from build123d import *

# Parameters (mm, degrees)
SKETCH_1_R          = 70
SKETCH_1_R_2        = 58
EXTRUDE_1_DEPTH     = 9
SKETCH_3_R          = 70
SKETCH_3_R_2        = 61
CUT_EXTRUDE_2_DEPTH = 3
CUT_EXTRUDE_3_DEPTH = 100.403219264
FILLET_1_R          = 10
CUT_EXTRUDE_6_DEPTH = 97.044388064
FILLET_7_R          = 3
SKETCH_6_R          = 1.5
CUT_EXTRUDE_4_DEPTH = 10
FILLET_9_R          = 5
EXTRUDE_START       = -1
SKETCH_9_R          = 58
SKETCH_9_R_2        = 56
EXTRUDE_2_DEPTH     = 1


with BuildPart() as part:
    # 草图1 → 凸台-拉伸1 (new body)
    with BuildSketch(Plane(origin=(0, 0, 0), x_dir=(1, 0, 0), z_dir=(0, 1, 0))):
        with Locations(Location((0, 0, 0), (0, 0, 270))):
            Circle(SKETCH_1_R)
        with Locations(Location((0, 0, 0), (0, 0, 270))):
            Circle(SKETCH_1_R_2, mode=Mode.SUBTRACT)
    extrude(amount=EXTRUDE_1_DEPTH)

    # 草图3 → 切除-拉伸2 (cut)
    with BuildSketch(Plane.XZ):
        with Locations(Location((0, 0, 0), (0, 0, 270))):
            Circle(SKETCH_3_R)
        with Locations(Location((0, 0, 0), (0, 0, 270))):
            Circle(SKETCH_3_R_2, mode=Mode.SUBTRACT)
    extrude(amount=-CUT_EXTRUDE_2_DEPTH, mode=Mode.SUBTRACT)

    # 草图4 → 切除-拉伸3 (cut, through all)
    with BuildSketch(Plane(origin=(0, 9, 0), x_dir=(1, 0, 0), z_dir=(0, 1, 0))):
        with BuildLine():
            Line((35.848527272, 51.197002768), (40.150350545, 57.3406431))
            ThreePointArc((40.150350545, 57.3406431), (0, 70), (-40.150350545, 57.3406431))
            Line((-40.150350545, 57.3406431), (-35.848527272, 51.197002768))
            ThreePointArc((-35.848527272, 51.197002768), (0, 62.5), (35.848527272, 51.197002768))
        make_face()
        with BuildLine():
            Line((51.197002768, 35.848527272), (57.3406431, 40.150350545))
            ThreePointArc((57.3406431, 40.150350545), (68.936542711, 12.155372437), (67.61480784, -18.117333157))
            Line((67.61480784, -18.117333157), (60.370364143, -16.176190319))
            ThreePointArc((60.370364143, -16.176190319), (61.550484563, 10.853011104), (51.197002768, 35.848527272))
        make_face()
        with BuildLine():
            Line((16.176190319, -60.370364143), (18.117333157, -67.61480784))
            ThreePointArc((18.117333157, -67.61480784), (-12.155372437, -68.936542711), (-40.150350545, -57.3406431))
            Line((-40.150350545, -57.3406431), (-35.848527272, -51.197002768))
            ThreePointArc((-35.848527272, -51.197002768), (-10.853011104, -61.550484563), (16.176190319, -60.370364143))
        make_face()
        with BuildLine():
            Line((-51.197002768, -35.848527272), (-57.3406431, -40.150350545))
            ThreePointArc((-57.3406431, -40.150350545), (-70, 0), (-57.3406431, 40.150350545))
            Line((-57.3406431, 40.150350545), (-51.197002768, 35.848527272))
            ThreePointArc((-51.197002768, 35.848527272), (-62.5, 0), (-51.197002768, -35.848527272))
        make_face()
    extrude(amount=-CUT_EXTRUDE_3_DEPTH, mode=Mode.SUBTRACT)

    # 圆角1
    # the kernel refuses this fillet: 10 mm, written as the material it adds along each edge
    with BuildSketch(Plane(origin=(-51.197002768, 9, 35.848527272), x_dir=(-0.8191520442890221, 0, 0.5735764363510029), z_dir=(0, -1, 0)), Plane(origin=(51.197002768, 9, -35.848527272), x_dir=(0.8191520442890228, 0, -0.5735764363510018), z_dir=(0, -1, 0)), Plane(origin=(-35.848527272, 9, -51.197002768), x_dir=(-0.5735764363510008, 0, -0.8191520442890236), z_dir=(0, -1, 0))) as fillet_1_piece_1:
        with BuildLine():
            CenterArc((9.330357143, 9.831062645), FILLET_1_R, 187.793366371, 71.660001872)
            Line((-0.577278325, 8.475054004), (-0.775431034, 8.447933831))
            ThreePointArc((-0.775431034, 8.447933831), (-0.344024235, 4.233754448), (-0.2, 0))
            Line((-0.2, 0), (0, -0.2))
            ThreePointArc((0, -0.2), (3.75, -0.2), (7.463392857, -0.196621253))
            Line((7.463392857, -0.196621253), (7.5, 0))
        make_face()
    extrude(amount=6)
    with BuildSketch(Plane(origin=(-35.848527272, 9, 51.197002768), x_dir=(-0.5735764363510476, 0, 0.8191520442889907), z_dir=(0, -1, 0))) as fillet_1_piece_2:
        with BuildLine():
            CenterArc((9.330357143, -9.831062645), FILLET_1_R, 100.546631757, 71.660001872)
            Line((-0.577278325, -8.475054004), (-0.775431034, -8.447933831))
            ThreePointArc((-0.775431034, -8.447933831), (-0.344024235, -4.233754448), (-0.2, 0))
            Line((-0.2, 0), (0, 0.2))
            ThreePointArc((0, 0.2), (3.75, 0.2), (7.463392857, 0.196621253))
            Line((7.463392857, 0.196621253), (7.5, 0))
        make_face()
    extrude(amount=6)
    with BuildSketch(Plane(origin=(35.848527272, 9, -51.197002768), x_dir=(-0.8562371813975653, 0, -0.5165828967284464), z_dir=(0, -1, 0)), Plane(origin=(-51.197002768, 9, -35.848527272), x_dir=(-0.5165828967284464, 0, 0.8562371813975653), z_dir=(0, -1, 0))) as fillet_1_piece_3:
        with BuildLine():
            CenterArc((9.174267262, 9.976882145), FILLET_1_R, 194.443314943, 71.660001872)
            Line((-0.509681515, 7.482661609), (-0.70336049, 7.432777198))
            ThreePointArc((-0.70336049, 7.432777198), (-0.4543784, 3.727739297), (-0.199537643, -0.013591507))
            Line((-0.199537643, -0.013591507), (0.013591507, -0.199537643))
            ThreePointArc((0.013591507, -0.199537643), (4.247345955, -0.055513408), (8.481100403, -0.199537643))
            Line((8.481100403, -0.199537643), (8.49469191, 0))
        make_face()
    extrude(amount=6)

    # 草图8 → 切除-拉伸6 (cut, through all)
    with BuildSketch(Plane(origin=(0, 9, 0), x_dir=(1, 0, 0), z_dir=(0, 1, 0))):
        with BuildLine():
            Line((26.62495049, -57.097390583), (29.583278322, -63.441545093))
            ThreePointArc((29.583278322, -63.441545093), (49.497474683, -49.497474683), (63.441545093, -29.583278322))
            Line((63.441545093, -29.583278322), (57.097390583, -26.62495049))
            ThreePointArc((57.097390583, -26.62495049), (44.547727215, -44.547727215), (26.62495049, -57.097390583))
        make_face()
    extrude(amount=-CUT_EXTRUDE_6_DEPTH, mode=Mode.SUBTRACT)

    # 圆角7
    fillet_7_edges = [part.edges().sort_by_distance(p)[0] for p in [
        (26.62495049, 6, 57.097390583),
        (57.097390583, 6, 26.62495049),
        (60.370364143, 6, 16.176190319),
        (16.176190319, 6, 60.370364143),
    ]]
    fillet(fillet_7_edges, radius=FILLET_7_R)

    # 草图6 → 切除-拉伸4 (cut)
    with BuildSketch(Plane(origin=(0, 9, 0), x_dir=(1, 0, 0), z_dir=(0, 1, 0))):
        with Locations(Location((42.423982239, 50.558933246, 0), (0, 0, 270))):
            Circle(SKETCH_6_R)
        with Locations(Location((-42.423982239, -50.558933246, 0), (0, 0, 270))):
            Circle(SKETCH_6_R)
        with Locations(Location((-50.558933246, 42.423982239, 0), (0, 0, 270))):
            Circle(SKETCH_6_R)
        with Locations(Location((50.558933246, 42.423982239, 0), (0, 0, 90))):
            Circle(SKETCH_6_R)
        with Locations(Location((-50.558933246, -42.423982239, 0), (0, 0, 90))):
            Circle(SKETCH_6_R)
        with Locations(Location((-42.423982239, 50.558933246, 0), (0, 0, 90))):
            Circle(SKETCH_6_R)
        with Locations(Location((22.573329459, -62.019712972, 0), (0, 0, 270))):
            Circle(SKETCH_6_R)
        with Locations(Location((62.019712972, -22.573329459, 0), (0, 0, 90))):
            Circle(SKETCH_6_R)
    extrude(amount=-CUT_EXTRUDE_4_DEPTH, mode=Mode.SUBTRACT)

    # 圆角9
    fillet_9_edges = [part.edges().sort_by_distance(p)[0] for p in [
        (67.61480784, 6, 18.117333157),
        (63.441545093, 6, 29.583278322),
        (18.117333157, 6, 67.61480784),
        (29.583278322, 6, 63.441545093),
    ]]
    fillet(fillet_9_edges, radius=FILLET_9_R)

    # 草图9 → 凸台-拉伸2 (add)
    with BuildSketch(Plane(origin=(0, 9, 0), x_dir=(1, 0, 0), z_dir=(0, 1, 0)).offset(EXTRUDE_START)):
        with Locations(Location((0, 0, 0), (0, 0, 270))):
            Circle(SKETCH_9_R)
        with Locations(Location((0, 0, 0), (0, 0, 270))):
            Circle(SKETCH_9_R_2, mode=Mode.SUBTRACT)
    extrude(amount=EXTRUDE_2_DEPTH)


solid = part.part
The listing builds one solid part. Answer for the finished solid, in the listing's coordinates (mm). A direction names the side the tool comes from. Round coordinates to 2 decimals unless told otherwise and drop trailing zeros. Order: outer loops, then holes, each group sorted by start corner. A loop starts at its lowest first (then second) coordinate and runs counter-clockwise, first axis right, second up. Notation, with made-up numbers: (26, 29.25) -> (66, 29.25) arc R7 cw to (66, 41.25) -> close; hole circle Ø3 at (54.5, 4). An arc over 180 degrees is marked (long way). One line per item, written item: value.
Item 1: Find section B-B, the plane z = 0. Give the vertices of the cut face in (x, y).
Taken from the geometry:
outline: (-62.5, 3) -> (-61, 3) -> (-61, 0) -> (-58, 0) -> (-58, 8) -> (-56, 8) -> (-56, 9) -> (-62.5, 9) -> close; (56, 8) -> (58, 8) -> (58, 0) -> (61, 0) -> (61, 3) -> (62.5, 3) -> (62.5, 9) -> (56, 9) -> close
Item 2: Given P1, Ø5, axis at x = 42.42, z = -50.56, coming from the -Y side; P2, Ø2, axis at y = 5, z = 31.5, coming from the -X side; P3, Ø1.8, axis at x = -50.56, z = 42.42, coming from the +Y side; P4, Ø4, axis at x = -19, y = 6, coming from the +Z side, each flat-ended and moving along its own axis, determine where each tip first touches the part or whether it passes through.
Taken from the geometry:
P1: stops at y = 3
P2: stops at x = -54.84
P3: passes through
P4: stops at z = 60.14
Item 3: For a pull along X with two mould halves and no side action, classify faces 1 (the cylindrical face through (-62.5, 6, -0.4)), 2 (the flat face through (-22, 0, 54)), 3 (the cylindrical face through (40.96, 6.04, -50.88)) as released by +X, released by -X, zero draft, split by the parting line, or undercut.
Taken from the geometry:
face 1: released by -X
face 2: zero draft
face 3: undercut
Item 4: Straight lines are drawn through the part: L1, parallel to Z at x = 1, y = 1; L2, parallel to Y at x = 51.5, z = -38; L3, parallel to X at y = 6.5, z = -21. For each, find the intervals that lie inside material, in ascending order.
Taken from the geometry:
L1: z = -60.99 to -57.99, 57.99 to 60.99
L2: y = 3 to 9
L3: x = -58.87 to -54.06, 54.06 to 58.87
Item 5: Find section A-A, the plane x = 0. Give the vertices of the cut face in (y, z).
Taken from the geometry:
outline: (0, -61) -> (3, -61) -> (3, -62.5) -> (9, -62.5) -> (9, -56) -> (8, -56) -> (8, -58) -> (0, -58) -> close; (0, 58) -> (8, 58) -> (8, 56) -> (9, 56) -> (9, 62.5) -> (3, 62.5) -> (3, 61) -> (0, 61) -> close
Item 6: For faces 4 (the cylindrical face through (-43.34, 6.04, 49.37)), 5 (the flat face through (50, 3, 36)), determine the directions among +Z, -Z, +X, -X, +Y, -Y from which every point of the face is accessible in a straight line to the end or side of a thin tool.
Taken from the geometry:
face 4: +Y, -Y
face 5: -Y
